```python
from build123d import *

# Parameters (mm, degrees)
BOSS_EXTRUDE1_DEPTH     = 10
CUT_EXTRUDE1_DEPTH      = 44.588989435
CUT_EXTRUDE1_DEPTH_BACK = 44.588989435
SKETCH2_R               = 2
CUT_EXTRUDE2_DEPTH      = 44.588989435
CUT_EXTRUDE2_DEPTH_BACK = 44.588989435
SKETCH3_R               = 2
CUT_EXTRUDE3_START      = -2
SKETCH4_W               = 27
SKETCH4_H               = 8
CUT_EXTRUDE3_DEPTH      = 42.588989435
CUT_EXTRUDE5_DEPTH      = 44.588989435
CUT_EXTRUDE5_DEPTH_BACK = 44.588989435
FILLET1_R               = 2
CUT_EXTRUDE6_DEPTH      = 44.588989435
CUT_EXTRUDE6_DEPTH_BACK = 44.588989435
SKETCH7_R               = 1.5


with BuildPart() as part:
    # Sketch1 → Boss-Extrude1 (new body)
    with BuildSketch(Plane.XY):
        Polygon((0, 0), (0, 30), (30, 0), align=None)
    extrude(amount=BOSS_EXTRUDE1_DEPTH)

    # Sketch2 → Cut-Extrude1 (cut, two sides: drawn at the far end of the back side and taken through both)
    with BuildSketch(Plane.ZY.offset(-CUT_EXTRUDE1_DEPTH_BACK)):
        with Locations(Location((5, 23, 0), (0, 0, 90))):
            Circle(SKETCH2_R)
        with Locations(Location((5, 10, 0), (0, 0, 90))):
            Circle(SKETCH2_R)
    extrude(amount=CUT_EXTRUDE1_DEPTH + CUT_EXTRUDE1_DEPTH_BACK, mode=Mode.SUBTRACT)

    # Sketch3 → Cut-Extrude2 (cut, two sides: drawn at the far end of the back side and taken through both)
    with BuildSketch(Plane.XZ.offset(-CUT_EXTRUDE2_DEPTH_BACK)):
        with Locations(Location((23, 5, 0), (0, 0, 138.590377891))):
            Circle(SKETCH3_R)
        with Locations(Location((10, 5, 0), (0, 0, 90))):
            Circle(SKETCH3_R)
    extrude(amount=CUT_EXTRUDE2_DEPTH + CUT_EXTRUDE2_DEPTH_BACK, mode=Mode.SUBTRACT)

    # Sketch4 → Cut-Extrude3 (cut, through all)
    with BuildSketch(Plane.XZ.offset(CUT_EXTRUDE3_START)):
        with Locations((15.5, 5)):
            Rectangle(SKETCH4_W, SKETCH4_H)
    extrude(amount=-CUT_EXTRUDE3_DEPTH, mode=Mode.SUBTRACT)

    # Sketch6 → Cut-Extrude5 (cut, two sides: drawn at the far end of the back side and taken through both)
    with BuildSketch(Plane(origin=(0, 0, 0), x_dir=(-1, 0, 0), z_dir=(0, 0, -1)).offset(-CUT_EXTRUDE5_DEPTH_BACK)):
        Polygon((-25.171572875, 2), (-15.719669914, 11.451902961), (-15.719669914, 2), align=None)
        Polygon((-2, 25.171572875), (-2, 15.719669914), (-11.451902961, 15.719669914), align=None)
        Polygon((-3.767766953, 2), (-13.219669914, 2), (-13.219669914, 11.451902961), align=None)
        Polygon((-2, 3.767766953), (-11.451902961, 13.219669914), (-2, 13.219669914), align=None)
    extrude(amount=CUT_EXTRUDE5_DEPTH + CUT_EXTRUDE5_DEPTH_BACK, mode=Mode.SUBTRACT)

    # Fillet1
    fillet1_edges = [part.edges().sort_by_distance(p)[0] for p in [
        (2, 13.219669914, 0.5),
        (2, 13.219669914, 9.5),
        (2, 3.767766953, 0.5),
        (2, 3.767766953, 9.5),
        (11.451902961, 13.219669914, 0.5),
        (11.451902961, 13.219669914, 9.5),
        (3.767766953, 2, 0.5),
        (3.767766953, 2, 9.5),
        (13.219669914, 11.451902961, 0.5),
        (13.219669914, 11.451902961, 9.5),
        (13.219669914, 2, 0.5),
        (13.219669914, 2, 9.5),
        (2, 25.171572875, 0.5),
        (2, 25.171572875, 9.5),
        (11.451902961, 15.719669914, 0.5),
        (11.451902961, 15.719669914, 9.5),
        (2, 15.719669914, 0.5),
        (2, 15.719669914, 9.5),
        (0, 0, 5),
        (15.719669914, 2, 0.5),
        (15.719669914, 2, 9.5),
        (25.171572875, 2, 0.5),
        (25.171572875, 2, 9.5),
        (15.719669914, 11.451902961, 0.5),
        (15.719669914, 11.451902961, 9.5),
    ]]
    fillet(fillet1_edges, radius=FILLET1_R)

    # Sketch7 → Cut-Extrude6 (cut, two sides: drawn at the far end of the back side and taken through both)
    with BuildSketch(Plane(origin=(0, 0, 0), x_dir=(-1, 0, 0), z_dir=(0, 0, -1)).offset(-CUT_EXTRUDE6_DEPTH_BACK)):
        with Locations((-12.525126266, 12.525126266)):
            Circle(SKETCH7_R)
    extrude(amount=CUT_EXTRUDE6_DEPTH + CUT_EXTRUDE6_DEPTH_BACK, mode=Mode.SUBTRACT)


solid = part.part
```
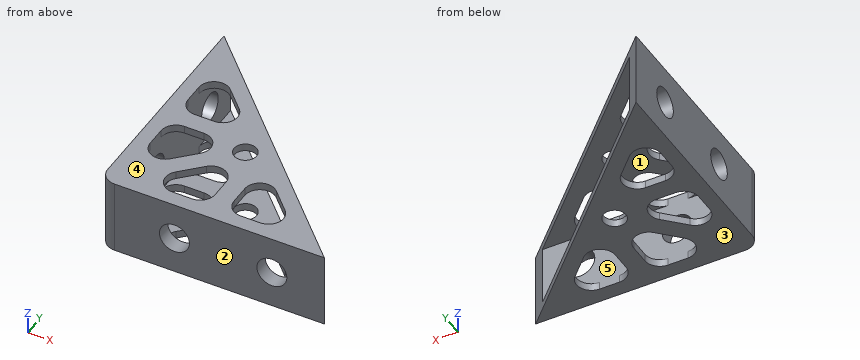
Check sheet for the modelled part. Datum: model origin and axes. Units: mm. Face numbers are marked on the shaded views. A direction names the side the tool comes from. Coordinates: 2 decimals unless noted, no trailing zeros. Order: outer loops, then holes, each group sorted by start corner. A loop starts at its lowest first (then second) coordinate and runs counter-clockwise, first axis right, second up. Notation, with made-up numbers: (5.5, 41.5) -> (49.5, 41.5) arc R33 cw to (49.5, 73.5) -> close; hole circle Ø8 at (13.5, 60). An arc over 180 degrees is marked (long way). Write item = value, one per line. Start each with the question number.
1) Cross-section at C-C (z = 5). Enter the section's corners in (x, y), then the cut area to 3 significant figures.
2) Material ranges on L1, parallel to Z at x = 14.5, y = 4; L2, parallel to Z at x = 1, y = 10; L3, parallel to X at y = 6, z = 8.5, recorded low to high.
3) Cross-section at B-B (x = 17). Enter the section's corners in (y, z).
4) Go/stop test with flat-tipped pins: P1, Ø3, axis at x = 7.5, z = 7, coming from the +Y side; P2, Ø1.1, axis at x = 5, z = 0.5, coming from the +Y side; P3, Ø3, axis at y = 8.5, z = 6.5, coming from the +X side; P4, Ø3, axis at x = 10, z = 5, coming from the +Y side. Record where each tip stops, or that it passes through.
5) Mould release check, pull along Z, two halves, no side actions. Record for the marked faces 3, 4 and 5: +Z half, -Z half, draft (parallel to the pull), parting line (faces both ways), or undercut.
6) Access from +Z, -Z, +X, -X, +Y, -Y to the whole of each face (thin tool, end or side, straight path). Record for the marked faces 1 and 2.
7) Cross-section at A-A (y = 23). Enter the section's corners in (x, z), then the cut area to 3 significant figures.
Ans:
q1.outline = (0, 2) arc R2 ccw to (2, 0) -> (8, 0) -> (8, 2) -> (2, 2) -> (2, 8) -> (0, 8) -> close; (0, 12) -> (2, 12) -> (2, 21) -> (0, 21) -> close; (0, 25) -> (2, 25) -> (2, 28) -> (0, 30) -> close; (12, 0) -> (21, 0) -> (21, 2) -> (12, 2) -> close; (25, 0) -> (30, 0) -> (28, 2) -> (25, 2) -> close
q1.area = 79.1 mm²
q2.L1 = 0 to 1, 9 to 10
q2.L2 = 0 to 3, 7 to 10
q2.L3 = 0 to 2
q3.outline = (0, 0) -> (2.13, 0) -> (2.13, 1) -> (2, 1) -> (2, 9) -> (2.13, 9) -> (2.13, 10) -> (0, 10) -> close; (8.49, 0) -> (13, 0) -> (13, 1) -> (8.49, 1) -> close; (8.49, 9) -> (13, 9) -> (13, 10) -> (8.49, 10) -> close
q4.P1 = 2
q4.P2 = 25.55
q4.P3 = 2
q4.P4 = through
q5.face_3 = -Z half
q5.face_4 = +Z half
q5.face_5 = undercut
q6.face_1 = +X, +Y
q6.face_2 = +Z, -Z, +X, -X, -Y
q7.outline = (0, 0) -> (7, 0) -> (7, 1) -> (2, 1) -> (2, 3) -> (0, 3) -> close; (0, 7) -> (2, 7) -> (2, 9) -> (7, 9) -> (7, 10) -> (0, 10) -> close
q7.area = 22.0 mm²
